```python
from build123d import *

# Parameters (mm, degrees)
ESQUISSE1_W          = 60
ESQUISSE1_H          = 25
ESQUISSE1_R          = 3.975
BASE_EXTRUSION_DEPTH = 19
ESQUISSE2_W          = 7
ESQUISSE2_H          = 34.447811935


with BuildPart() as part:
    # Esquisse1 → Base-Extrusion (new body)
    with BuildSketch(Plane.XY):
        with Locations((0, -6.5)):
            Rectangle(ESQUISSE1_W, ESQUISSE1_H)
        with Locations((-20, 0)):
            Circle(ESQUISSE1_R, mode=Mode.SUBTRACT)
        with Locations(Location((0, 0, 0), (0, 0, 180))):
            Circle(ESQUISSE1_R, mode=Mode.SUBTRACT)
        with Locations((20, 0)):
            Circle(ESQUISSE1_R, mode=Mode.SUBTRACT)
    extrude(amount=BASE_EXTRUSION_DEPTH)

    # Esquisse2 → Enlever de la matière-Révolution2 (revolve, cut)
    with BuildSketch(Plane(origin=(0, 0, 0), x_dir=(0, 0, -1), z_dir=(0.9945218953682731, -0.10452846326765709, 0)), mode=Mode.PRIVATE) as enlever_de_la_mati_re_r_volution2_sk:
        with Locations((-6.059329615, -6.776094032)):
            Rectangle(ESQUISSE2_W, ESQUISSE2_H)
    revolve(enlever_de_la_mati_re_r_volution2_sk.sketch.rotate(Axis((0.951521061, 9.053118164, 9.559329615), (-0.10452846326765709, -0.994521895368273, 0)), 90), axis=Axis((0.951521061, 9.053118164, 9.559329615), (-0.10452846326765709, -0.994521895368273, 0)), mode=Mode.SUBTRACT)


solid = part.part
```
The listing builds one solid part. Answer for the finished solid, in the listing's coordinates (mm). Coordinates: 2 decimals unless noted, no trailing zeros. Loops run counter-clockwise (first coordinate to the right, second up) from the corner with the lowest first, then second, coordinate; pieces in that order, holes last. Notation, with made-up numbers: (-31, 34) - (-1, 34) arc R15 ccw to (-1, 44) - close; hole circle Ø5 at (-17, -28.75). An arc over 180 degrees is marked (long way). Use a Markdown table: item, result. Add a question column.
1) The mould has two halves that part along X. Classify faces 1 (the cylindrical face through (-3.672, 1.522, 1.45)), 2 (the flat face through (-7, 6, 9)), 3 (the flat face through (30, -7, 9)): released by +X, released by -X, zero draft, split by the parting line, or undercut.
2) Find the intervals of material crossed by line 1 (Y direction, x = 20, z = 5.75) (3 decimals); line 2 (X direction, y = 0.75, z = 8); line 3 (X direction, y = -0.5, z = 3), in increasing order.
3) The part is cut by section A-A, the plane x = -20. Give the vertices of the cut face in (y, z) (3 decimals).
4) The part is cut by section C-C, the plane y = 2.25. State how many separate pieces and enclosed holes the cut face has, and give its area (3 significant figures).
5) The part is cut by section D-D, the plane x = 21.5. Give the vertices of the cut face in (y, z).
6) The part is cut by section B-B, the plane z = 7. Give the vertices of the cut face in (x, y) (3 decimals), and give its area (3 significant figures).
Here are the results:
| question | item | result |
|---|---|---|
| 1 | face 1 | undercut |
| 1 | face 2 | zero draft |
| 1 | face 3 | released by +X |
| 2 | line 1 | y = -19 to -3.975, 3.975 to 6 |
| 2 | line 2 | x = -30 to -23.9, -16.1 to -6.78, 6.94 to 16.1, 23.9 to 30 |
| 2 | line 3 | x = -30 to -23.94, -16.06 to -3.94, 3.94 to 16.06, 23.94 to 30 |
| 3 | outline | (-19, 0) - (-3.975, 0) - (-3.975, 19) - (-19, 19) - close; (3.975, 0) - (6, 0) - (6, 19) - (3.975, 19) - close |
| 4 | separate pieces | 4 |
| 4 | enclosed holes | 0 |
| 4 | area | 700 mm^2 |
| 5 | outline | (-19, 0) - (-3.68, 0) - (-3.68, 19) - (-19, 19) - close; (3.68, 0) - (6, 0) - (6, 19) - (3.68, 19) - close |
| 6 | outline | (-30, -19) - (-8.548, -19) - (-5.921, 6) - (-30, 6) - close; (4.554, -19) - (30, -19) - (30, 6) - (7.182, 6) - close; hole circle Ø7.95 at (-20, 0); hole circle Ø7.95 at (20, 0) |
| 6 | area | 1,070 mm^2 |
